```python
from build123d import *

# Parameters (mm, degrees)
SKETCH2_W            = 22.86
SKETCH2_H            = 12.7
BOSS_EXTRUDE1_DEPTH  = 0.8
SKETCH3_R            = 0.4
CUT_EXTRUDE1_DEPTH   = 14.172979921
LPATTERN1_COUNT      = 10
LPATTERN1_PITCH      = 2.54
LPATTERN1_COUNT_DIR2 = 6
LPATTERN1_PITCH_DIR2 = 2.54


with BuildPart() as part:
    # Sketch2 → Boss-Extrude1 (new, symmetric)
    with BuildSketch(Plane(origin=(0, 0, 0), x_dir=(1, 0, 0), z_dir=(0, 1, 0))):
        Rectangle(SKETCH2_W, SKETCH2_H)
    extrude(amount=BOSS_EXTRUDE1_DEPTH, both=True)

    # Sketch3 → Cut-Extrude1 (cut, through all)
    with BuildSketch(Plane(origin=(0, 0.8, 0), x_dir=(1, 0, 0), z_dir=(0, 1, 0))):
        with Locations((-11.43, 6.35)):
            Circle(SKETCH3_R)
    cut_extrude1 = extrude(amount=-CUT_EXTRUDE1_DEPTH, mode=Mode.SUBTRACT)

    # LPattern1: Cut-Extrude1 10 × 6
    with Locations(*[(i * LPATTERN1_PITCH, 0, j * LPATTERN1_PITCH_DIR2) for i in range(LPATTERN1_COUNT) for j in range(LPATTERN1_COUNT_DIR2) if (i, j) != (0, 0)]):
        add(cut_extrude1, mode=Mode.SUBTRACT)


solid = part.part
```
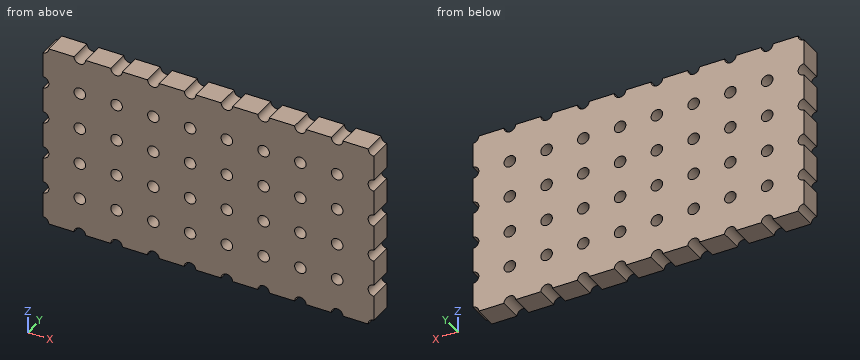
Geometry check sheet. Reference: the model listing, model coordinates, mm. Round coordinates to 2 decimals unless told otherwise and drop trailing zeros. Write each loop counter-clockwise with the first axis right and the second up, starting at its lowest first coordinate (ties: lowest second). Pieces come first, ordered by that corner, then holes. Notation, with made-up numbers: (46, 67) -> (75, 67) arc R27 ccw to (75, 88) -> close; hole circle Ø1 at (-19.75, 49.5). An arc over 180 degrees is marked (long way). Put each result on its own line as item: value.
1) Cross-section at A-A, the plane x = 8.89. Enter the section's corners in (y, z), plus the area to 3 significant figures.
Recorded:
outline: (-0.8, -5.95) -> (0.8, -5.95) -> (0.8, -4.21) -> (-0.8, -4.21) -> close; (-0.8, -3.41) -> (0.8, -3.41) -> (0.8, -1.67) -> (-0.8, -1.67) -> close; (-0.8, -0.87) -> (0.8, -0.87) -> (0.8, 0.87) -> (-0.8, 0.87) -> close; (-0.8, 1.67) -> (0.8, 1.67) -> (0.8, 3.41) -> (-0.8, 3.41) -> close; (-0.8, 4.21) -> (0.8, 4.21) -> (0.8, 5.95) -> (-0.8, 5.95) -> close
area: 13.9 mm2
2) Thickness scan on probe 1 along Z at (x, y) = (1.27, -0.25); probe 2 along Z at (x, y) = (-6, 0). Record the ranges inside material, lowest first. Write a range as from..to.
Recorded:
probe 1: z = -5.95..-4.21, -3.41..-1.67, -0.87..0.87, 1.67..3.41, 4.21..5.95
probe 2: z = -6.16..-4, -3.62..-1.46, -1.08..1.08, 1.46..3.62, 4..6.16
3) Cross-section at B-B, the plane z = 3.81. Give the number of separate pieces and of enclosed holes in the cut face, plus the area to 3 significant figures.
Recorded:
separate pieces: 9
enclosed holes: 0
area: 25.1 mm2
